The model under review builds one solid part; all positions refer to its coordinate system, in mm. A direction names the side the tool comes from. Coordinates: 2 decimals unless noted, no trailing zeros. Write each loop counter-clockwise with the first axis right and the second up, starting at its lowest first coordinate (ties: lowest second). Pieces come first, ordered by that corner, then holes.
```python
from build123d import *

# Parameters (mm, degrees)
SM_BASE_FLANGE_1_DEPTH = 1
OTHER_1_DEPTH          = 70
OTHER_START            = 25
OTHER_1_2_DEPTH        = 20
OTHER_1_3_DEPTH        = 15
OTHER_START_2          = 55
OTHER_1_4_DEPTH        = 15
SKETCH_12_R            = 2
CUT_EXTRUDE_1_DEPTH    = 10
OTHER_START_3          = -1
OTHER_1_5_DEPTH        = 1
FILLET_1_R             = 0.25
FILLET_2_R             = 5


# Read off the part's stored shape, not the designer's step: 햄1, 코너 자르기1
# Sheet-metal steps are written as plain solids
with BuildPart() as part:
    # Sketch 1 → 베이스-플랜지1 (new body)
    with BuildSketch(Plane.XY):
        Polygon((0, 0), (0, 25), (15, 25), (15, 20), (25, 20), (25, 25), (45, 25), (45, 20), (55, 20), (55, 25), (70, 25), (70, 0), align=None)
    extrude(amount=-SM_BASE_FLANGE_1_DEPTH)

    # Other 1 outline → Other 1 (cut)
    with BuildSketch(Plane.YZ):
        with BuildLine():
            ThreePointArc((23, 0), (24, -0.267949192), (24.732050807, -1))
            Line((24.732050807, -1), (25, -1))
            Line((25, -1), (25, 0))
            Line((25, 0), (23, 0))
        make_face()
    extrude(amount=OTHER_1_DEPTH, mode=Mode.SUBTRACT)

    # Other 1 2 outline → Other 1 2 (add)
    with BuildSketch(Plane.YZ.offset(OTHER_START)):
        with BuildLine():
            Line((22.015192247, -1.826351822), (21.030384494, -1.652703645))
            ThreePointArc((21.030384494, -1.652703645), (23.347296355, -3.969615506), (24.732050807, -1))
            Line((24.732050807, -1), (23, -1))
            ThreePointArc((23, -1), (23.64278761, -2.766044443), (22.015192247, -1.826351822))
        make_face()
    extrude(amount=OTHER_1_2_DEPTH)

    # Other 1 3 outline → Other 1 3 (add)
    with BuildSketch(Plane.YZ):
        with BuildLine():
            Line((22.015192247, -1.826351822), (21.030384494, -1.652703645))
            ThreePointArc((21.030384494, -1.652703645), (23.347296355, -3.969615506), (24.732050807, -1))
            Line((24.732050807, -1), (23, -1))
            ThreePointArc((23, -1), (23.64278761, -2.766044443), (22.015192247, -1.826351822))
        make_face()
    extrude(amount=OTHER_1_3_DEPTH)

    # Other 1 4 outline → Other 1 4 (add)
    with BuildSketch(Plane.YZ.offset(OTHER_START_2)):
        with BuildLine():
            Line((22.015192247, -1.826351822), (21.030384494, -1.652703645))
            ThreePointArc((21.030384494, -1.652703645), (23.347296355, -3.969615506), (24.732050807, -1))
            Line((24.732050807, -1), (23, -1))
            ThreePointArc((23, -1), (23.64278761, -2.766044443), (22.015192247, -1.826351822))
        make_face()
    extrude(amount=OTHER_1_4_DEPTH)

    # 스케치12 → 컷-돌출1 (cut)
    with BuildSketch(Plane(origin=(0, 0, -1), x_dir=(-1, 0, 0), z_dir=(0, 0, -1))):
        with Locations((-35, 10)):
            Circle(SKETCH_12_R)
        with Locations((-55, 10)):
            Circle(SKETCH_12_R)
        with Locations((-15, 10)):
            Circle(SKETCH_12_R)
    extrude(amount=-CUT_EXTRUDE_1_DEPTH, mode=Mode.SUBTRACT)

    # Other 1 5 outline → Other 1 5 (add)
    with BuildSketch(Plane.XY.offset(OTHER_START_3)):
        with BuildLine():
            Line((45, 20), (45.25, 20))
            ThreePointArc((45.25, 20), (45.073223305, 20.073223305), (45, 20.25))
            Line((45, 20.25), (45, 20))
        make_face()
        with BuildLine():
            ThreePointArc((55, 20.25), (54.926776695, 20.073223305), (54.75, 20))
            Line((54.75, 20), (55, 20))
            Line((55, 20), (55, 20.25))
        make_face()
    extrude(amount=OTHER_1_5_DEPTH)

    # 필렛1
    fillet_1_edges = [part.edges().sort_by_distance(p)[0] for p in [
        (15, 20, -0.5),
        (25, 20, -0.5),
    ]]
    fillet(fillet_1_edges, radius=FILLET_1_R)

    # 필렛2
    fillet_2_edges = [part.edges().sort_by_distance(p)[0] for p in [
        (0, 0, -0.5),
        (70, 0, -0.5),
    ]]
    fillet(fillet_2_edges, radius=FILLET_2_R)


solid = part.part
```
Item 1: Take a section at B-B, the plane y = 10. Write out the cut boundary in (x, z), plus the area to 3 significant figures.
Solved:
outline: (0, -1) - (13, -1) - (13, 0) - (0, 0) - close; (17, -1) - (33, -1) - (33, 0) - (17, 0) - close; (37, -1) - (53, -1) - (53, 0) - (37, 0) - close; (57, -1) - (70, -1) - (70, 0) - (57, 0) - close
area: 58.0 mm2
Item 2: For pin 1 (6.5 mm diameter, centred on x = 55, y = 10, fed in from -Z); pin 2 (0.5 mm diameter, centred on x = 49, z = -0.5, fed in from +Y), all flat-tipped, find the tip position at first contact; note any pin that passes through.
Solved:
pin 1: stops at z = -1
pin 2: stops at y = 20
Item 3: To check wall thickness, follow line 1 along X through (y, z) = (22.5, -0.4); line 2 along Y through (x, z) = (37, -2); line 3 along X through (y, z) = (11, -0.65). State the ranges of each line that lie inside material, in increasing order.
Solved:
line 1: x = 0 to 15, 25 to 45, 55 to 70
line 2: y = 21 to 22, 24 to 25
line 3: x = 0 to 13.27, 16.73 to 33.27, 36.73 to 53.27, 56.73 to 70
Item 4: Mouldability with a two-part tool opening along X and no side actions: class faces 3 (the face through (62.4, 23.67, -2.74)), 4 (the face through (25, 24, -1)), 5 (the face through (70, 16.4, -0.7)) as pulls with the +X half, pulls with the -X half, needs draft (parallel to the pull), parting line crosses it, or undercut.
Solved:
face 3: needs draft
face 4: undercut
face 5: pulls with the +X half
Item 5: Take a section at D-D, the plane y = 16. Write out the cut boundary in (x, z), plus the area to 3 significant figures.
Solved:
outline: (0, -1) - (70, -1) - (70, 0) - (0, 0) - close
area: 70.0 mm2
Item 6: Take a section at A-A, the plane x = 35. Write out the cut boundary in (y, z), plus the area to 3 significant figures.
Solved:
outline: (0, -1) - (8, -1) - (8, 0) - (0, 0) - close; (12, -1) - (23, -1) arc R1 cw (long way) to (22.02, -1.83) - (21.03, -1.65) arc R2 ccw (long way) to (23, 0) - (12, 0) - close
area: 26.3 mm2
Item 7: Take a section at C-C, the plane x = 28. Write out the cut boundary in (y, z), plus the area to 3 significant figures.
Solved:
outline: (0, -1) - (23, -1) arc R1 cw (long way) to (22.02, -1.83) - (21.03, -1.65) arc R2 ccw (long way) to (23, 0) - (0, 0) - close
area: 30.3 mm2
Item 8: Machinability: for faces 1 (the face through (7.4, 23.67, -2.74)), 2 (the face through (45, 24, -1)), which of the approach directions +Z, -Z, +X, -X, +Y, -Y give a long, thin tool a straight path to every point of the face, cutting with its end or side? Answer none if there is none.
Solved:
face 1: +X, -X
face 2: +Z, -Z, +Y
